CAD build for the part. Positions are in the model's coordinates, mm. A direction names the side the tool comes from. Coordinates: 2 decimals unless noted, no trailing zeros. Loops run counter-clockwise (first coordinate to the right, second up) from the corner with the lowest first, then second, coordinate; pieces in that order, holes last. Notation, with made-up numbers: M 78.25,49.5 L 113.25,49.5 A27 ccw 113.25,74.5 Z; hole C 82.5,-5 d11. An arc over 180 degrees is marked long. Answer as a JSON object with one key per item and string values. Group by question number.
```python
from build123d import *

# Parameters (mm, degrees)
SKETCH1_R           = 3.15
BOSS_EXTRUDE1_DEPTH = 7.5
SKETCH2_W           = 4
SKETCH2_H           = 4
BOSS_EXTRUDE2_DEPTH = 2.5
CUT_EXTRUDE1_START  = -7.5
SKETCH3_W           = 3
SKETCH3_H           = 13
CUT_EXTRUDE1_DEPTH  = 6
SKETCH4_W           = 3
SKETCH4_H           = 13
CUT_EXTRUDE2_DEPTH  = 6
SKETCH5_W           = 26
SKETCH5_H           = 3
CUT_EXTRUDE3_DEPTH  = 6
BOSS_EXTRUDE3_DEPTH = 5.9


with BuildPart() as part:
    # Sketch1 → Boss-Extrude1 (new, symmetric)
    with BuildSketch(Plane.XY):
        Polygon((-30, -5), (-30, 8), (30, 8), (30, -5), (24, -5), (24, 6), (14, 6), (14, -5), align=None)
        with Locations((-19, 0)):
            Circle(SKETCH1_R, mode=Mode.SUBTRACT)
        Circle(SKETCH1_R, mode=Mode.SUBTRACT)
    extrude(amount=BOSS_EXTRUDE1_DEPTH, both=True)

    # Sketch2 → Boss-Extrude2 (add)
    with BuildSketch(Plane.XZ.offset(5)):
        with Locations((8, 0)):
            Rectangle(SKETCH2_W, SKETCH2_H)
        with Locations((-8, 0)):
            Rectangle(SKETCH2_W, SKETCH2_H)
    extrude(amount=BOSS_EXTRUDE2_DEPTH)

    # Sketch3 → Cut-Extrude1 (cut)
    with BuildSketch(Plane.XY.offset(CUT_EXTRUDE1_START)):
        with Locations((-28.5, 1.5)):
            Rectangle(SKETCH3_W, SKETCH3_H)
        with Locations((28.5, 1.5)):
            Rectangle(SKETCH3_W, SKETCH3_H)
    extrude(amount=CUT_EXTRUDE1_DEPTH, mode=Mode.SUBTRACT)

    # Sketch4 → Cut-Extrude2 (cut)
    with BuildSketch(Plane.XY.offset(7.5)):
        with Locations((28.5, 1.5)):
            Rectangle(SKETCH4_W, SKETCH4_H)
        with Locations((-28.5, 1.5)):
            Rectangle(SKETCH4_W, SKETCH4_H)
    extrude(amount=-CUT_EXTRUDE2_DEPTH, mode=Mode.SUBTRACT)

    # Sketch5 → Cut-Extrude3 (cut)
    with BuildSketch(Plane(origin=(0, 0, -7.5), x_dir=(-1, 0, 0), z_dir=(0, 0, -1))):
        with Locations((0, 6.5)):
            Rectangle(SKETCH5_W, SKETCH5_H)
    extrude(amount=-CUT_EXTRUDE3_DEPTH, mode=Mode.SUBTRACT)

    # Sketch6 → Boss-Extrude3 (add)
    with BuildSketch(Plane(origin=(0, 0, -7.5), x_dir=(-1, 0, 0), z_dir=(0, 0, -1))):
        with BuildLine():
            Line((-14, 6), (-17.9, 6))
            ThreePointArc((-17.9, 6), (-15.702704612, 5.132040834), (-14, 3.494281042))
            Line((-14, 3.494281042), (-14, 6))
        make_face()
        with BuildLine():
            Line((-24, 6), (-24, 3.494281042))
            ThreePointArc((-24, 3.494281042), (-22.297295388, 5.132040834), (-20.1, 6))
            Line((-20.1, 6), (-24, 6))
        make_face()
    extrude(amount=-BOSS_EXTRUDE3_DEPTH)


solid = part.part
```
Item 1: Pin check, flat tips, straight feed: pin 1 (2 mm diameter, centred on x = 15.5, y = 4.5, fed in from +Z); pin 2 (3 mm diameter, centred on y = -0.5, z = -4, fed in from -X); pin 3 (1.5 mm diameter, centred on x = -28.5, y = 4, fed in from -Z). Stop position of each tip, or through.
Item 2: Tool access for faces 4 (the flat face through (14, 1, 0)), 5 (the flat face through (13, 6, -5)), 6 (the flat face through (28, 2, 1.5)): list every direction of +Z, -Z, +X, -X, +Y, -Y with a clear straight run to the whole face (end or side of a thin tool).
Item 3: Drill centre lines: L1, parallel to Y at x = -19, z = 4.75; L2, parallel to Y at x = 0, z = -3.75; L3, parallel to X at y = 1.25, z = 6.5. Where is each one in solid material? Low to high. Write a range as from..to.
Item 4: Slice it at A-A, the plane z = -6. Write the cut outline in (x, y).
Item 5: Pull direction X, two halves, no side cores. Call faces 1 (the flat face through (30, 2, 0)), 2 (the flat face through (-6, -6, 0)), 3 (the flat face through (-29, 2, -1.5)): released by +X, released by -X, zero draft, split by the parting line, or undercut.
Item 6: Slice it at B-B, the plane x = -19. Write the cut outline in (y, z).
Item 7: Slice it at C-C, the plane y = -6. Write the cut outline in (x, z), then the cut area to 3 significant figures.
Item 8: Slice it at D-D, the plane y = 0. Write the cut outline in (x, z).
Computed:
{
 "1": {"pin 1": "z = -1.6", "pin 2": "x = -27", "pin 3": "z = -1.5"},
 "2": {"face 4": "+Z, -Y", "face 5": "-Z, +Y", "face 6": "+Z, +X, +Y, -Y"},
 "3": {"L1": "-5..-3.15, 3.15..8", "L2": "-5..-3.15, 3.15..5", "L3": "-27..-21.89, -16.11..-2.89, 2.89..14, 24..27"},
 "4": {"outline": "M -27,-5 L 14,-5 L 14,3.49 A6.1 cw 17.9,6 L 20.1,6 A6.1 cw 24,3.49 L 24,-5 L 27,-5 L 27,8 L 13,8 L 13,5 L -13,5 L -13,8 L -27,8 Z; hole C -19,0 d6.3; hole C 0,0 d6.3"},
 "5": {"face 1": "released by +X", "face 2": "undercut", "face 3": "zero draft"},
 "6": {"outline": "M -5,-7.5 L -3.15,-7.5 L -3.15,7.5 L -5,7.5 Z; M 3.15,-7.5 L 8,-7.5 L 8,7.5 L 3.15,7.5 Z"},
 "7": {"outline": "M -10,-2 L -6,-2 L -6,2 L -10,2 Z; M 6,-2 L 10,-2 L 10,2 L 6,2 Z", "area": "32.0 mm2"},
 "8": {"outline": "M -30,-1.5 L -27,-1.5 L -27,-7.5 L -22.15,-7.5 L -22.15,7.5 L -27,7.5 L -27,1.5 L -30,1.5 Z; M -15.85,-7.5 L -3.15,-7.5 L -3.15,7.5 L -15.85,7.5 Z; M 3.15,-7.5 L 14,-7.5 L 14,7.5 L 3.15,7.5 Z; M 24,-7.5 L 27,-7.5 L 27,-1.5 L 30,-1.5 L 30,1.5 L 27,1.5 L 27,7.5 L 24,7.5 Z"}
}
